Verification items for this drawing (mm, ordinates from the low corner). A direction names the side the tool comes from. Give positions to 0.01 mm unless a question says otherwise; leave off trailing zeros. Loops run counter-clockwise (first coordinate to the right, second up) from the corner with the lowest first, then second, coordinate; pieces in that order, holes last. Notation, with made-up numbers: M 44.5,-33.75 L 83.5,-33.75 A18 cw 83.5,-5.75 Z; hole C -18.5,28.5 d6. An arc over 180 degrees is marked long. Use a Markdown table: item, result.
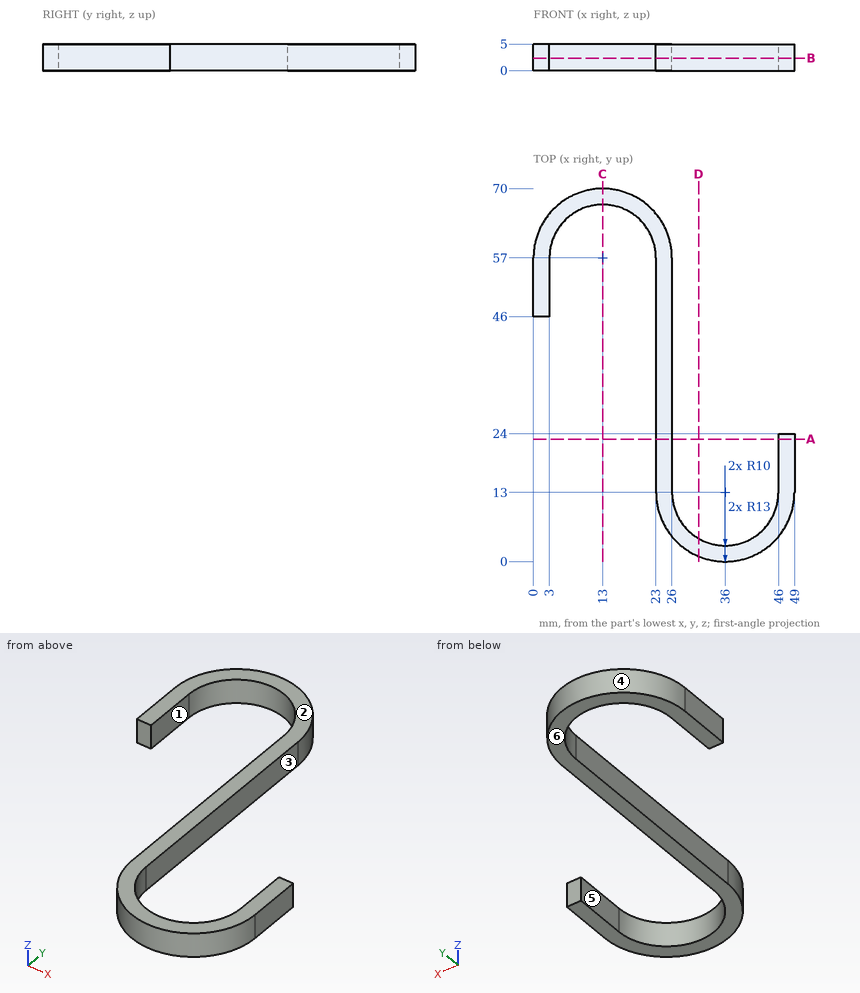
(1) Cross-section at B-B on z = 2.35. Record the cut outline in (x, y), then the cut area to 3 significant figures.
Results below:
| item | result |
|---|---|
| outline | M 0,46 L 3,46 L 3,57 A10 cw 23,57 L 23,13 A13 ccw 49,13 L 49,24 L 46,24 L 46,13 A10 cw 26,13 L 26,57 A13 ccw 0,57 Z |
| area | 415 mm^2 |
(2) Cross-section at D-D on x = 31. Record the cut outline in (y, z).
Results below:
| item | result |
|---|---|
| outline | M 1,0 L 4.34,0 L 4.34,5 L 1,5 Z |
(3) Cross-section at A-A on y = 23. Record the cut outline in (x, z).
Results below:
| item | result |
|---|---|
| outline | M 23,0 L 26,0 L 26,5 L 23,5 Z; M 46,0 L 49,0 L 49,5 L 46,5 Z |
(4) Draft check along X on the marked faces 3, 4, 5 and 6. Enter one of: +X half, -X half, draft (parallel to the pull), parting line (faces both ways), or undercut.
Results below:
| item | result |
|---|---|
| face 3 | undercut |
| face 4 | parting line |
| face 5 | undercut |
| face 6 | draft |
(5) Set-up check for the marked faces 1 and 2: record each of +Z, -Z, +X, -X, +Y, -Y from which the full face is reachable in a straight line by a thin tool's end or side.
Results below:
| item | result |
|---|---|
| face 1 | +Z, -Z, -Y |
| face 2 | +Z, +X, -X, +Y, -Y |
(6) Gauge pin test, flat ends, axial feed: P1, Ø1.5, axis at y = 19.5, z = 3.5, coming from the -X side; P2, Ø0.9, axis at x = 48, z = 2, coming from the +Y side; P3, Ø2.5, axis at y = 52, z = 3, coming from the +X side. Record the tip position at first contact, or that the pin passes through.
Results below:
| item | result |
|---|---|
| P1 | x = 23 |
| P2 | y = 24 |
| P3 | x = 26 |
(7) Material ranges on line 1 (X direction, y = 18.5, z = 0.7); line 2 (X direction, y = 50, z = 1); line 3 (X direction, y = 44, z = 1), recorded low to high.
Results below:
| item | result |
|---|---|
| line 1 | 23 to 26, 46 to 49 |
| line 2 | 0 to 3, 23 to 26 |
| line 3 | 23 to 26 |
(8) Cross-section at C-C on x = 13. Record the cut outline in (y, z).
Results below:
| item | result |
|---|---|
| outline | M 67,0 L 70,0 L 70,5 L 67,5 Z |
